Design review of the part built by this model. Coordinates are the model's own, in mm. A direction names the side the tool comes from. Coordinates: 2 decimals unless noted, no trailing zeros.
Q1. Machinability: for faces 5 (the face through (1, 44, 19)), 6 (the face through (31, 6, -25)), 7 (the face through (-32, 6, 25)), 8 (the face through (1.671, 51.349, 37.963)), which of the approach directions +Z, -Z, +X, -X, +Y, -Y give a long, thin tool a straight path to every point of the face, cutting with its end or side? Answer none if there is none.
Q2. To check wall thickness, follow probe 1 along X at (y, z) = (27, 33); probe 2 along X at (y, z) = (31, 0); probe 3 along X at (y, z) = (35.5, 25.5). State the ranges of each line that lie inside material, in increasing order.
Q3. The part is to be moulded in two halves that separate along Y. For faces 1 (the face through (12, 66.8, 38)), 2 (the face through (-32, 6, -25)), 3 (the face through (38, 82.7, -12)), 4 (the face through (38.547, 20.773, 0.378)), say which applies: +Y half, -Y half, draft (parallel to the pull), parting line (faces both ways), or undercut.
Q4. Clearance check with flat-ended pins moving along their axes: pin 1 Ø6 at (x, y) = (22.5, 71.5) entering from -Z; pin 2 Ø6 at (x, z) = (30.5, -12.5) entering from +Y; pin 3 Ø1.7 at (x, y) = (32.5, 4.5) entering from +Z. State where each tip first meets the part, or that it passes through.
Q5. Add section B-B, the plane z = 21. Give the number of separate pieces and of enclosed holes in the cut face, plus the area to 3 significant figures.
from build123d import *

# Parameters (mm, degrees)
KUBBE1_FACE_RADIUS          = 42.5
KUBBE1_HEIGHT               = 5
KES_EKSTR_ZYON1_DEPTH       = 113.41663578
KES_EKSTR_ZYON1_DEPTH_BACK  = 113.41663578
IZIM2_R                     = 16.9
IZIM3_R                     = 38
KES_EKSTR_ZYON3_DEPTH       = 85
KES_EKSTR_ZYON4_DEPTH       = 113.416635855
KES_EKSTR_ZYON4_DEPTH_BACK  = 113.416635855
Y_KSEKLIK_EKSTR_ZYON1_START = 19
IZIM5_R                     = 22.5
Y_KSEKLIK_EKSTR_ZYON1_DEPTH = 19
Y_KSEKLIK_EKSTR_ZYON1_TAPER = 16
Y_KSEKLIK_EKSTR_ZYON2_START = -19
IZIM9_R                     = 22.5
Y_KSEKLIK_EKSTR_ZYON2_DEPTH = 19
Y_KSEKLIK_EKSTR_ZYON2_DRAFT = -16
KES_EKSTR_ZYON6_DEPTH       = 132.573173651
KES_EKSTR_ZYON6_DEPTH_BACK  = 132.573173651
IZIM10_R                    = 16.9


with BuildPart() as part:
    # Çizim1 → Döndür1 (revolve)
    with BuildSketch(Plane.XY, mode=Mode.PRIVATE) as d_nd_r1_sk:
        Polygon((0, 0), (0, 90), (42.5, 90), (42.5, 82.7), (39.5, 82.7), (39.5, 78.4), (42.5, 78.4), (42.5, 71.1), (39.5, 71.1), (39.5, 66.8), (42.5, 66.8), (42.5, 59.5), (39.5, 59.5), (39.5, 55.2), (42.5, 55.2), (42.5, 0), align=None)
    revolve(d_nd_r1_sk.sketch.rotate(Axis((0, 0, 0), (0, 1, 0)), 90), axis=Axis((0, 0, 0), (0, 1, 0)))

    # Kubbe1: a dome of height H over a round flat face of radius A is a cap of a sphere of radius (A * A + H * H) / (2 * H)
    kubbe1_r = (KUBBE1_FACE_RADIUS * KUBBE1_FACE_RADIUS + KUBBE1_HEIGHT * KUBBE1_HEIGHT) / (2 * KUBBE1_HEIGHT)
    kubbe1_base = Plane((0, 90, 0), z_dir=(0, 1, 0))
    with Locations(kubbe1_base.offset(KUBBE1_HEIGHT - kubbe1_r)):
        kubbe1_ball = Sphere(kubbe1_r, mode=Mode.PRIVATE)
    add(split(kubbe1_ball, bisect_by=kubbe1_base, keep=Keep.TOP, mode=Mode.PRIVATE))

    # Çizim2 → Kes-Ekstrüzyon1 (cut, two sides: drawn at the far end of the back side and taken through both)
    with BuildSketch(Plane.XY.offset(-KES_EKSTR_ZYON1_DEPTH_BACK)):
        with Locations((-2.119743269, 27)):
            Circle(IZIM2_R)
    extrude(amount=KES_EKSTR_ZYON1_DEPTH + KES_EKSTR_ZYON1_DEPTH_BACK, mode=Mode.SUBTRACT)

    # Çizim3 → Kes-Ekstrüzyon3 (cut)
    with BuildSketch(Plane(origin=(0, 0, 0), x_dir=(-1, 0, 0), z_dir=(0, -1, 0))):
        with Locations(Location((0, 0, 0), (0, 0, 90))):
            Circle(IZIM3_R)
    extrude(amount=-KES_EKSTR_ZYON3_DEPTH, mode=Mode.SUBTRACT)

    # Çizim4 → Kes-Ekstrüzyon4 (cut, two sides: drawn at the far end of the back side and taken through both)
    with BuildSketch(Plane(origin=(0, 0, 0), x_dir=(0, 0, -1), z_dir=(1, 0, 0)).offset(-KES_EKSTR_ZYON4_DEPTH_BACK)):
        with BuildLine():
            Line((-25, 0), (-25, 12))
            ThreePointArc((-25, 12), (0, 20.775010008), (25, 12))
            Line((25, 12), (25, 0))
            Line((25, 0), (-25, 0))
        make_face()
    extrude(amount=KES_EKSTR_ZYON4_DEPTH + KES_EKSTR_ZYON4_DEPTH_BACK, mode=Mode.SUBTRACT)

    # Çizim5 → Yükseklik-Ekstrüzyon1 (add)
    with BuildSketch(Plane.XY.offset(Y_KSEKLIK_EKSTR_ZYON1_START)):
        with Locations((-2.119743269, 27)):
            Circle(IZIM5_R)
    extrude(amount=Y_KSEKLIK_EKSTR_ZYON1_DEPTH, taper=Y_KSEKLIK_EKSTR_ZYON1_TAPER)


with BuildPart() as y_kseklik_ekstr_zyon2_tool:
    # Çizim9 → Yükseklik-Ekstrüzyon2 (with draft: the straight prism first)
    with BuildSketch(Plane.XY.offset(Y_KSEKLIK_EKSTR_ZYON2_START)):
        with Locations((-2.119743269, 27)):
            Circle(IZIM9_R)
    extrude(amount=-Y_KSEKLIK_EKSTR_ZYON2_DEPTH)
    # Yükseklik-Ekstrüzyon2: the draft: its side faces are tilted about the plane it starts from
    y_kseklik_ekstr_zyon2_sides = [y_kseklik_ekstr_zyon2_tool.faces().sort_by_distance(p)[0] for p in [
        (-24.619743269, 27, -28.5),
    ]]
    draft(y_kseklik_ekstr_zyon2_sides, Plane.XY.offset(Y_KSEKLIK_EKSTR_ZYON2_START), Y_KSEKLIK_EKSTR_ZYON2_DRAFT)


with BuildPart() as part_1:
    add(part.part)

    # Yükseklik-Ekstrüzyon2: add y_kseklik_ekstr_zyon2_tool
    add(y_kseklik_ekstr_zyon2_tool.part)

    # Çizim10 → Kes-Ekstrüzyon6 (cut, two sides: drawn at the far end of the back side and taken through both)
    with BuildSketch(Plane(origin=(0, 0, -38), x_dir=(-1, 0, 0), z_dir=(0, 0, -1)).offset(-KES_EKSTR_ZYON6_DEPTH_BACK)):
        with Locations(Location((2.119743269, 27, 0), (0, 0, 180))):
            Circle(IZIM10_R)
    extrude(amount=KES_EKSTR_ZYON6_DEPTH + KES_EKSTR_ZYON6_DEPTH_BACK, mode=Mode.SUBTRACT)


solid = part_1.part
Here are the results:
1. face 5: -Y
1. face 6: +X, -Y
1. face 7: -X, -Y
1. face 8: none
2. probe 1: x = -26.78 to -19.02, 14.78 to 16.37, 18.84 to 26.78
2. probe 2: x = -42.5 to -38, 38 to 42.5
2. probe 3: x = -34 to -28.17, -20.92 to -16.73, 12.49 to 16.68, 28.17 to 34
3. face 1: undercut
3. face 2: draft
3. face 3: undercut
3. face 4: -Y half
4. pin 1: stops at z = -37.76
4. pin 2: stops at y = 92.53
4. pin 3: stops at z = 28.36
5. separate pieces: 2
5. enclosed holes: 1
5. area: 1,820 mm2
